Answer from the drawing. Dimensions are ordinates in mm from the lowest x, y and z of the part. A direction names the side the tool comes from. Round coordinates to 2 decimals unless told otherwise and drop trailing zeros. Write each loop counter-clockwise with the first axis right and the second up, starting at its lowest first coordinate (ties: lowest second). Pieces come first, ordered by that corner, then holes. Notation, with made-up numbers: (20, -30.75) - (25, -30.75) arc R22 cw to (25, 8.25) - close; hole circle Ø8 at (21.5, -30). An arc over 180 degrees is marked (long way). Write item = value, one per line. Start each with the question number.
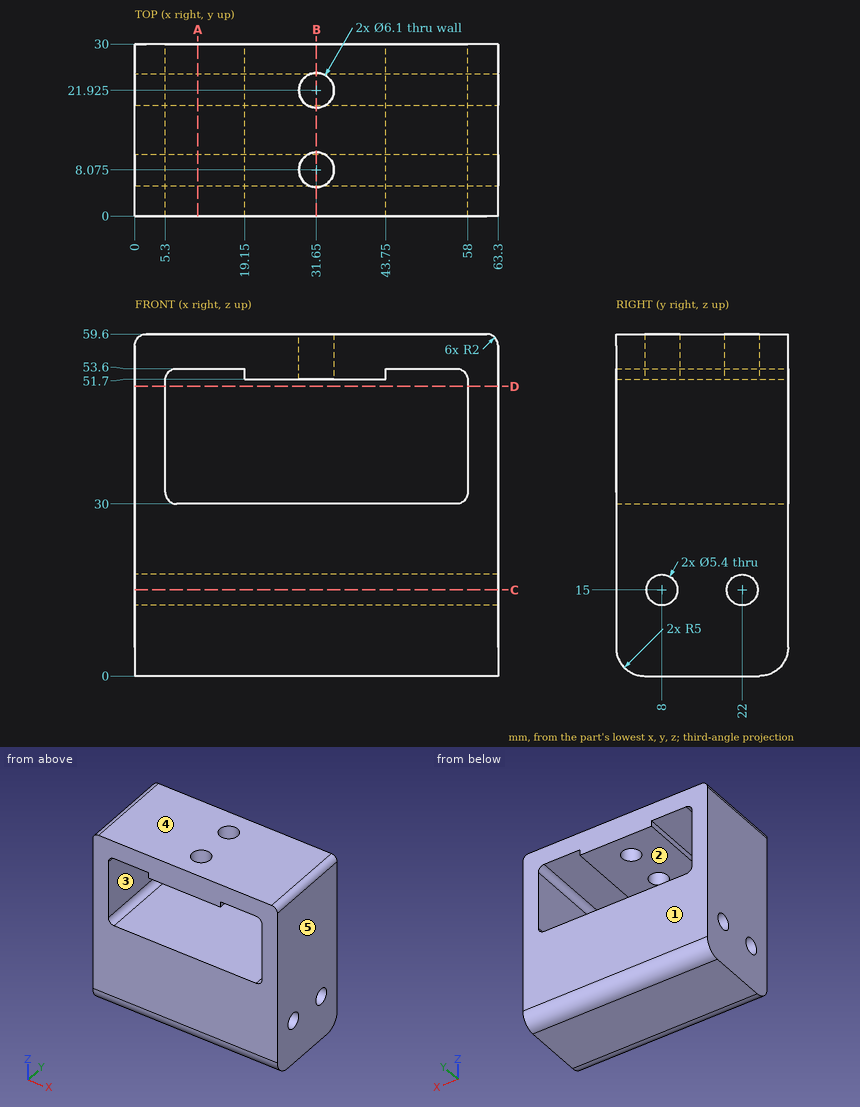
1. Which of the six approach directions +Z, -Z, +X, -X, +Y, -Y give full straight-line access (tool end or side, diameter ignored) to the marked faces 1 and 2?
2. Find section D-D on z = 50.5. Give the vertices of the cut face in (x, y).
3. Find section C-C on z = 15. Give the vertices of the cut face in (x, y).
4. Find section B-B on x = 31.65. Give the vertices of the cut face in (y, z) (3 decimals).
5. Consider line 1 (Z direction, x = 7.5, y = 22); line 2 (Z direction, x = 35, y = 8); line 3 (Y direction, x = 31.65, z = 55.25) (3 decimals). Determine where each line is inside the solid, lowest interval first.
6. Find section A-A on x = 11. Give the vertices of the cut face in (y, z), plus the area to 3 significant figures.
7. For a pull along Z with two mould halves and no side action, classify the marked faces 3, 4 and 5 as released by +Z, released by -Z, zero draft, split by the parting line, or undercut.
Answer key:
q1.face_1 = +Z, -Z, +X, -X, +Y
q1.face_2 = +Y, -Y
q2.outline = (0, 0) - (5.3, 0) - (5.3, 30) - (0, 30) - close; (58, 0) - (63.3, 0) - (63.3, 30) - (58, 30) - close
q3.outline = (0, 0) - (63.3, 0) - (63.3, 5.3) - (0, 5.3) - close; (0, 10.7) - (63.3, 10.7) - (63.3, 19.3) - (0, 19.3) - close; (0, 24.7) - (63.3, 24.7) - (63.3, 30) - (0, 30) - close
q4.outline = (0, 5) arc R5 ccw to (5, 0) - (25, 0) arc R5 ccw to (30, 5) - (30, 30) - (0, 30) - close; (0, 51.7) - (5.025, 51.7) - (5.025, 59.6) - (0, 59.6) - close; (11.125, 51.7) - (18.875, 51.7) - (18.875, 59.6) - (11.125, 59.6) - close; (24.975, 51.7) - (30, 51.7) - (30, 59.6) - (24.975, 59.6) - close; hole circle Ø5.4 at (8, 15); hole circle Ø5.4 at (22, 15)
q5.line_1 = 0 to 12.3, 17.7 to 30, 53.6 to 59.6
q5.line_2 = 0 to 12.3, 17.7 to 30, 51.7 to 59.6
q5.line_3 = 0 to 5.025, 11.125 to 18.875, 24.975 to 30
q6.outline = (0, 5) arc R5 ccw to (5, 0) - (25, 0) arc R5 ccw to (30, 5) - (30, 30) - (0, 30) - close; (0, 53.6) - (30, 53.6) - (30, 59.6) - (0, 59.6) - close; hole circle Ø5.4 at (8, 15); hole circle Ø5.4 at (22, 15)
q6.area = 1,020 mm²
q7.face_3 = undercut
q7.face_4 = released by +Z
q7.face_5 = zero draft
